The listing builds one solid part. Answer for the finished solid, in the listing's coordinates (mm). Face numbers are marked on the shaded views. Round coordinates to 2 decimals unless told otherwise and drop trailing zeros. Loops run counter-clockwise (first coordinate to the right, second up) from the corner with the lowest first, then second, coordinate; pieces in that order, holes last. Notation, with made-up numbers: (59.5, -9) -> (80.5, -9) arc R26 ccw to (80.5, 13) -> close; hole circle Ø9 at (-20.5, 32). An arc over 180 degrees is marked (long way). Use a Markdown table: item, result. Add a question column.
Q1. Consider line 1 (Z direction, x = -47, y = 9); line 2 (Y direction, x = 0, z = 1); line 3 (Y direction, x = -16, z = -7.5). Determine where each line is inside the solid, lowest interval first.
Q2. Section D-D on y = 96 is taken. Give the vertices of the cut face in (x, z).
Q3. Section A-A on z = 8.5 is taken. Give the vertices of the cut face in (x, y), then the cut area to 3 significant figures.
Q4. Section C-C on x = 0 is taken. Give the vertices of the cut face in (y, z).
Q5. For a pull along X with two mould halves and no side action, classify the marked faces 1 and 2 as released by +X, released by -X, zero draft, split by the parting line, or undercut.
Q6. Given pin 1 Ø8 at (x, z) = (-14, -7.5) entering from -Y; pin 2 Ø4.5 at (x, y) = (-51.5, -5) entering from -Z; pin 3 Ø5 at (y, z) = (117.5, -7.5) entering from +X, each flat-ended and moving along its own axis, determine where each tip first touches the part or whether it passes through.
Q7. Section B-B on y = 0 is taken. Give the vertices of the cut face in (x, z), then the cut area to 3 significant figures.
Solid Edge part; units mm, degrees
sketch "Sketch1" plane through (0, 0, 0) normal (0, 0, 1) x (1, 0, 0)
  line L0 (20, -125) -> (-20, -125)
  line L1 (-20, -125) -> (-20, 125)
  line L2 (-20, 125) -> (20, 125)
  line L3 (20, 125) -> (20, -125)
  circle A0 centre (0, 0) radius 10
  dimension "D1" = 20
  dimension "D2" = 20
extrude "Ajout_matière_1" add sketch "Sketch1" along normal blind 5
sketch "Sketch2" plane through (0, 0, 0) normal (0, 0, -1) x (0, 1, 0)
  line L0 (125, 10) -> (110, 10)
  line L1 (110, 10) -> (110, -10)
  line L2 (110, -10) -> (125, -10)
  line L3 (125, -10) -> (125, 10)
  dimension "D1" = 110
  dimension "D2" = 125
extrude "Enlèvement_matière_1" cut sketch "Sketch2" against normal blind 34.8434
sketch "Sketch3" plane through (0, 0, 0) normal (0, 0, -1) x (0, 1, 0)
  line L0 (125, -20) -> (110, -20)
  line L1 (110, -20) -> (110, -10)
  line L2 (110, -10) -> (125, -10)
  line L3 (125, -10) -> (125, -20)
  line L4 (125, 20) -> (110, 20)
  line L5 (110, 20) -> (110, 10)
  line L6 (110, 10) -> (125, 10)
  line L7 (125, 10) -> (125, 20)
extrude "Ajout_matière_2" add sketch "Sketch3" along normal blind 15
sketch "Sketch4" plane through (-20, 0, -5) normal (-1, 0, 0) x (0, 1, 0)
  circle A0 centre (117.5, 2.5) radius 2.0023
extrude "Enlèvement_matière_2" cut sketch "Sketch4" against normal blind 63.2944
fillet "Congé_1" radius 2 2 edges at (15, 110, 0) (-15, 110, 0)
sketch "Sketch5" plane through (-20, 0, -5) normal (-1, 0, 0) x (0, 1, 0)
  line L0 (-15, -10) -> (15, -10)
  line L1 (15, -10) -> (15, -5)
  line L2 (15, -5) -> (-15, -5)
  line L3 (-15, -5) -> (-15, -10)
  dimension "D1" = 15
extrude "Protrusion1" add sketch "Sketch5" along normal blind 39.7243
sketch "Sketch6" plane through (-19.8622, 0, 5) normal (0, 0, 1) x (0, -1, 0)
  line L0 (-15, -39.8622) -> (15, -39.8622)
  line L1 (15, -39.8622) -> (15, -33.8622)
  line L2 (15, -33.8622) -> (-15, -33.8622)
  line L3 (-15, -33.8622) -> (-15, -39.8622)
  dimension "D1" = 15
extrude "Ajout_matière_4" add sketch "Sketch6" along normal blind 12
sketch "Sketch7" plane through (-53.7243, 0, 11) normal (1, 0, 0) x (0, -1, 0)
  line L0 (-15, -6) -> (15, -6)
  line L1 (15, -6) -> (15, 0)
  line L2 (15, 0) -> (-15, 0)
  line L3 (-15, 0) -> (-15, -6)
extrude "Ajout_matière_7" add sketch "Sketch7" along normal blind 12
mirror "Mirror1" about plane through (0, 0, 0) normal (1, 0, 0) of "Ajout_matière_7", "Ajout_matière_4", "Protrusion1"
chamfer "Chanfrein_1" distance 3 angle 45 2 edges at (-41.7243, 0, 11) (41.7243, 0, 11)
properties material "Acier S235"
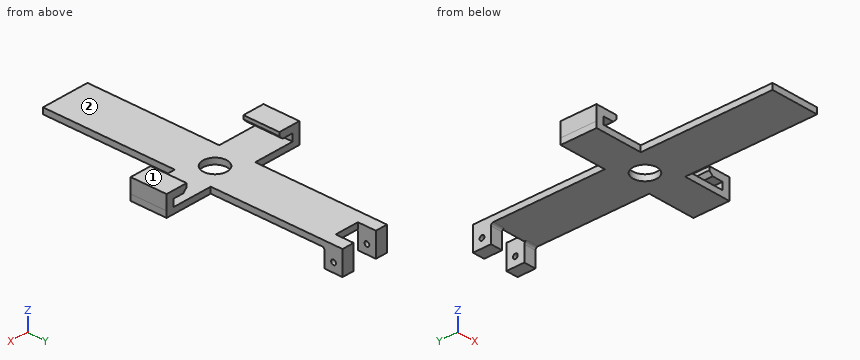
Checked values:
| question | item | result |
|---|---|---|
| 1 | line 1 | z = 0 to 5, 11 to 17 |
| 1 | line 2 | y = -125 to -10, 10 to 110 |
| 1 | line 3 | y = 110 to 115.5, 119.5 to 125 |
| 2 | outline | (-20, 0) -> (20, 0) -> (20, 5) -> (-20, 5) -> close |
| 3 | outline | (-59.72, -15) -> (-53.72, -15) -> (-53.72, 15) -> (-59.72, 15) -> close; (53.72, -15) -> (59.72, -15) -> (59.72, 15) -> (53.72, 15) -> close |
| 3 | area | 360 mm2 |
| 4 | outline | (-125, 0) -> (-10, 0) -> (-10, 5) -> (-125, 5) -> close; (10, 0) -> (110, 0) -> (110, 5) -> (10, 5) -> close |
| 5 | face 1 | zero draft |
| 5 | face 2 | undercut |
| 6 | pin 1 | stops at y = 110 |
| 6 | pin 2 | stops at z = 0 |
| 6 | pin 3 | stops at x = 20 |
| 7 | outline | (-59.72, 0) -> (-10, 0) -> (-10, 5) -> (-53.72, 5) -> (-53.72, 11) -> (-44.72, 11) -> (-41.72, 14) -> (-41.72, 17) -> (-59.72, 17) -> close; (10, 0) -> (59.72, 0) -> (59.72, 17) -> (41.72, 17) -> (41.72, 14) -> (44.72, 11) -> (53.72, 11) -> (53.72, 5) -> (10, 5) -> close |
| 7 | area | 776 mm2 |
